from build123d import *

# Parameters (mm, degrees)
SKETCH_1_R      = 2.5
SKETCH_1_R_2    = 5
EXTRUDE_1_DEPTH = 5


with BuildPart() as part:
    # 草圖1 → 填料-伸長1 (new body)
    with BuildSketch(Plane.XY):
        with BuildLine():
            Line((-42, -7), (0, -7))
            ThreePointArc((0, -7), (7, 0), (0, 7))
            Line((0, 7), (-42, 7))
            ThreePointArc((-42, 7), (-49, 0), (-42, -7))
        make_face()
        with Locations((-37.399198152, 0)):
            Circle(SKETCH_1_R, mode=Mode.SUBTRACT)
        Polygon((-21, 3.260013757), (-15.641541971, 0), (-21, -3.260013757), (-21, -1.630006879), (-28.07448836, -1.630006879), (-28.07448836, 1.630006879), (-21, 1.630006879), align=None, mode=Mode.SUBTRACT)
        with Locations((-4.031364092, 0)):
            Circle(SKETCH_1_R_2, mode=Mode.SUBTRACT)
    extrude(amount=EXTRUDE_1_DEPTH)


solid = part.part
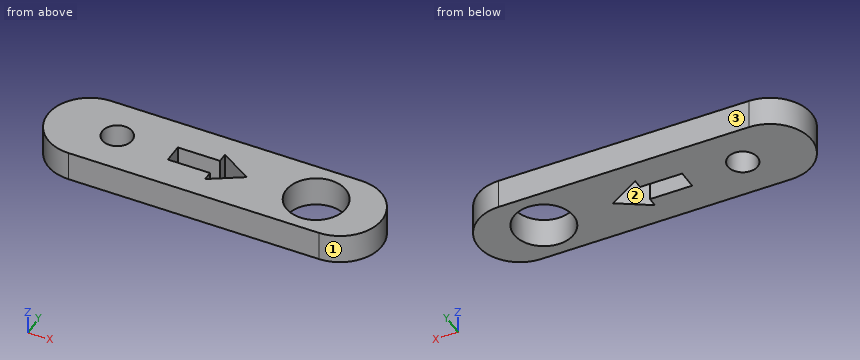
The model under review builds one solid part; all positions refer to its coordinate system, in mm. Face numbers are marked on the shaded views. Coordinates: 2 decimals unless noted, no trailing zeros. Loops run counter-clockwise (first coordinate to the right, second up) from the corner with the lowest first, then second, coordinate; pieces in that order, holes last. Notation, with made-up numbers: (22, -38.75) -> (62, -38.75) arc R18 ccw to (62, -14.75) -> close; hole circle Ø7 at (40, -15.5). An arc over 180 degrees is marked (long way). Use a Markdown table: item, result. Add a question column.
1. Clearance check with flat-ended pins moving along their axes: pin 1 Ø0.5 at (y, z) = (-2.5, 3.5) entering from +X; pin 2 Ø1.5 at (y, z) = (1, 3) entering from +X; pin 3 Ø0.8 at (y, z) = (2.5, 2) entering from +X; pin 4 Ø6 at (x, y) = (-37.4, 0) entering from +Z. State where each tip first meets the part, or that it passes through.
2. Add section D-D on y = 5.5. Write out the cut boundary in (x, z), plus the area to 3 significant figures.
3. Add section A-A on z = 3.2. Write out the cut boundary in (x, y).
4. Add section B-B on y = 0.75. Write out the cut boundary in (x, z), plus the area to 3 significant figures.
5. Draft analysis for pull direction Y (two halves, no side actions). For the marked faces 1, 2 and 3, state which applies: pulls with the +Y half, pulls with the -Y half, needs draft (parallel to the pull), parting line crosses it, or undercut.
6. Add section C-C on x = -5. Write out the cut boundary in (y, z).
7. To check wall thickness, follow line 1 (X direction, y = -0.75, z = 2); line 2 (Y direction, x = -4, z = 4.65); line 3 (X direction, y = -1.75, z = 1.6). State the ranges of each line that lie inside material, in increasing order.
Returned:
| question | item | result |
|---|---|---|
| 1 | pin 1 | stops at x = 6.63 |
| 1 | pin 2 | stops at x = 7 |
| 1 | pin 3 | stops at x = 6.68 |
| 1 | pin 4 | stops at z = 5 |
| 2 | outline | (-46.33, 0) -> (4.33, 0) -> (4.33, 5) -> (-46.33, 5) -> close |
| 2 | area | 253 mm² |
| 3 | outline | (-42, -7) -> (0, -7) arc R7 ccw to (0, 7) -> (-42, 7) arc R7 ccw to start; hole circle Ø5 at (-37.4, 0); hole (-28.07, -1.63) -> (-21, -1.63) -> (-21, -3.26) -> (-15.64, 0) -> (-21, 3.26) -> (-21, 1.63) -> (-28.07, 1.63) -> close; hole circle Ø10 at (-4.03, 0) |
| 4 | outline | (-48.96, 0) -> (-39.78, 0) -> (-39.78, 5) -> (-48.96, 5) -> close; (-35.01, 0) -> (-28.07, 0) -> (-28.07, 5) -> (-35.01, 5) -> close; (-16.87, 0) -> (-8.97, 0) -> (-8.97, 5) -> (-16.87, 5) -> close; (0.91, 0) -> (6.96, 0) -> (6.96, 5) -> (0.91, 5) -> close |
| 4 | area | 150 mm² |
| 5 | face 1 | parting line crosses it |
| 5 | face 2 | undercut |
| 5 | face 3 | pulls with the +Y half |
| 6 | outline | (-7, 0) -> (-4.91, 0) -> (-4.91, 5) -> (-7, 5) -> close; (4.91, 0) -> (7, 0) -> (7, 5) -> (4.91, 5) -> close |
| 7 | line 1 | x = -48.96 to -39.78, -35.01 to -28.07, -16.87 to -8.97, 0.91 to 6.96 |
| 7 | line 2 | y = -7 to -5, 5 to 7 |
| 7 | line 3 | x = -48.78 to -39.18, -35.61 to -21, -18.52 to -8.72, 0.65 to 6.78 |
